Can you work these out from the model? Positions are in its coordinate system, mm. Give positions to 0.01 mm unless a question says otherwise; leave off trailing zeros. Write each loop counter-clockwise with the first axis right and the second up, starting at its lowest first coordinate (ties: lowest second). Pieces come first, ordered by that corner, then holes.
1. Suppose I cut it at C-C (y = 11). Please give me the cut outline in (x, z), and give its area (3 significant figures).
2. Suppose I cut it at B-B (x = -26). Please give me the cut outline in (y, z), and give its area (3 significant figures).
3. If I drill on probe 1 along X at (y, z) = (8, 1.15); probe 2 along Y at (x, z) = (-9, 2.75); probe 3 along X at (y, z) = (7, 2.65), over which ranges is the centre line in solid material (lowest first)?
4. Suppose I cut it at A-A (z = 0.95). Please give me the cut outline in (x, y), and give its area (3 significant figures).
5. I'm going to push flat-ended pins straight in: pin 1 (1 mm diameter, centred on x = -29.5, z = 4, fed in from +Y); pin 2 (1 mm diameter, centred on x = -27, z = 3.5, fed in from +Y); pin 3 (1.5 mm diameter, centred on y = 42, z = 3.5, fed in from -X). Where does each tip first touch, or does it pass through?
6. Thinking about a two-plate mould opening in Y: for faces 1 (the cylindrical face through (-41.96, 42.89, 2.46)), 2 (the cylindrical face through (-45.397, 8.968, 2.535)), 3 (the flat face through (-26, 30, 5)), 4 (the flat face through (4.363, 30.69, 2.535)), which applies, pulls with the +Y half, pulls with the -Y half, needs draft (parallel to the pull), parting line crosses it, or undercut?
```python
from build123d import *

# Parameters (mm, degrees)
BOSS_EXTRUDE1_DEPTH = 5
SKETCH3_R           = 1.5
CUT_EXTRUDE1_DEPTH  = 5
BOSS_EXTRUDE2_DEPTH = 5


with BuildPart() as part:
    # Sketch2 → Boss-Extrude1 (new body)
    with BuildSketch(Plane.XY):
        with BuildLine():
            Line((-60, 0), (-14.999324285, -0.142376231))
            ThreePointArc((-14.999324285, -0.142376231), (-10.706799113, 10.505448717), (-0.142376231, 14.999324285))
            Line((-0.142376231, 14.999324285), (0, 60))
            ThreePointArc((0, 60), (-42.426406871, 42.426406871), (-60, 0))
        make_face()
    extrude(amount=BOSS_EXTRUDE1_DEPTH)

    # Sketch3 → Cut-Extrude1 (cut)
    with BuildSketch(Plane.XY.offset(5)):
        with Locations((-7.673918476, 44.34084996)):
            Circle(SKETCH3_R)
        with Locations((-44.291404204, 7.954339294)):
            Circle(SKETCH3_R)
    extrude(amount=-CUT_EXTRUDE1_DEPTH, mode=Mode.SUBTRACT)

    # Sketch4 → Boss-Extrude2 (add)
    with BuildSketch(Plane.XY.offset(5)):
        with BuildLine():
            Line((8.712482668, 35.840415418), (-0.109488527, 25.394099488))
            Line((-0.109488527, 25.394099488), (-0.056967441, 41.994372784))
            ThreePointArc((-0.056967441, 41.994372784), (4.465384672, 39.11351402), (8.712482668, 35.840415418))
        make_face()
    extrude(amount=-BOSS_EXTRUDE2_DEPTH)


solid = part.part
```
Checks:
1. outline: (-58.98, 0) - (-10.2, 0) - (-10.2, 5) - (-58.98, 5) - close
1. area: 244 mm2
2. outline: (-0.11, 0) - (54.07, 0) - (54.07, 5) - (-0.11, 5) - close
2. area: 271 mm2
3. probe 1: x = -59.46 to -45.79, -42.79 to -12.69
3. probe 2: y = 12 to 43.64, 45.04 to 59.32
3. probe 3: x = -59.59 to -45.45, -43.13 to -13.27
4. outline: (-60, 0) - (-15, -0.14) arc R15 cw to (-0.14, 15) - (-0.11, 25.39) - (8.71, 35.84) arc R60 ccw to (-0.06, 41.99) - (0, 60) arc R60 ccw to start; hole circle Ø3 at (-44.29, 7.95); hole circle Ø3 at (-7.67, 44.34)
4. area: 2,710 mm2
5. pin 1: stops at y = 52.53
5. pin 2: stops at y = 53.83
5. pin 3: stops at x = -43.57
6. face 1: pulls with the +Y half
6. face 2: undercut
6. face 3: needs draft
6. face 4: pulls with the -Y half
